Source: CAD feature listing. Evaluate the final solid. Frame: model axes, mm. A direction names the side the tool comes from. Round coordinates to 2 decimals unless told otherwise and drop trailing zeros. Write each loop counter-clockwise with the first axis right and the second up, starting at its lowest first coordinate (ties: lowest second). Pieces come first, ordered by that corner, then holes. Notation, with made-up numbers: M -22,-28.5 L -6,-28.5 A15 cw -6,-16.5 Z; hole C 88,49 d2. An arc over 180 degrees is marked long. Put each result on its own line as item: value. Start each with the question number.
```python
from build123d import *

# Parameters (mm, degrees)
SKETCH_1_R      = 1.7
EXTRUDE_1_DEPTH = 10
EXTRUDE_2_DEPTH = 1.3
FILLET_1_R      = 0.3
FILLET_2_R      = 0.3
SKETCH_3_R      = 1
EXTRUDE_3_DEPTH = 5
FILLET_3_R      = 2
SKETCH_4_W      = 3.4
SKETCH_4_H      = 10
EXTRUDE_4_DEPTH = 0.6


with BuildPart() as part:
    # 草圖1 → 填料-伸長1 (new body)
    with BuildSketch(Plane(origin=(0, 0, 0), x_dir=(1, 0, 0), z_dir=(0, 1, 0))):
        Polygon((13.5, -0.8), (11.5, -0.8), (11.5, -4.2), (13.5, -4.2), (13.5, -5), (0, -5), (-2.5, -5), (-2.5, 0), (0, 0), (13.5, 0), align=None)
        with Locations(Location((0, -2.5, 0), (0, 0, 270))):
            Circle(SKETCH_1_R, mode=Mode.SUBTRACT)
    extrude(amount=EXTRUDE_1_DEPTH)

    # 草圖2 → 填料-伸長2 (add)
    with BuildSketch(Plane(origin=(11.5, 0, 0), x_dir=(0, 0, -1), z_dir=(1, 0, 0))):
        Polygon((-4.2, 7.155796618), (-0.8, 5.655796618), (-0.8, 5), (-4.2, 6.5), align=None)
        Polygon((-4.2, 4.155796618), (-0.8, 2.655796618), (-0.8, 2), (-4.2, 3.5), align=None)
    extrude(amount=EXTRUDE_2_DEPTH)

    # 圓角1
    fillet_1_edges = [part.edges().sort_by_distance(p)[0] for p in [
        (12.8, 6.405796618, 2.5),
        (12.8, 5.75, 2.5),
        (12.8, 3.405796618, 2.5),
        (12.8, 2.75, 2.5),
    ]]
    fillet(fillet_1_edges, radius=FILLET_1_R - 0.0001)  # a hair under: the kernel refuses the full size

    # 圓角2
    fillet_2_edges = [part.edges().sort_by_distance(p)[0] for p in [
        (13.5, 5, 0),
        (13.5, 5, 0.8),
        (13.5, 5, 4.2),
        (13.5, 5, 5),
    ]]
    fillet(fillet_2_edges, radius=FILLET_2_R)

    # 草圖3 → 填料-伸長3 (add)
    with BuildSketch(Plane.XY):
        with BuildLine():
            Line((4.5, 10), (4.5, 15))
            ThreePointArc((4.5, 15), (7, 17.5), (9.5, 15))
            Line((9.5, 15), (9.5, 10))
            Line((9.5, 10), (4.5, 10))
        make_face()
        with Locations(Location((7, 15, 0), (0, 0, 180))):
            Circle(SKETCH_3_R, mode=Mode.SUBTRACT)
    extrude(amount=EXTRUDE_3_DEPTH)

    # 圓角3
    fillet_3_edges = [part.edges().sort_by_distance(p)[0] for p in [
        (-2.5, 5, 5),
        (-2.5, 5, 0),
    ]]
    fillet(fillet_3_edges, radius=FILLET_3_R)

    # 草圖4 → 填料-伸長4 (add)
    with BuildSketch(Plane(origin=(11.5, 0, 0), x_dir=(0, 0, -1), z_dir=(1, 0, 0))):
        with Locations((-2.5, 5)):
            Rectangle(SKETCH_4_W, SKETCH_4_H)
    extrude(amount=EXTRUDE_4_DEPTH)


solid = part.part
```
(1) Section query D-D (z = 3.55). Count the separate pieces of the cut face and the enclosed holes in it, and give its area (3 significant figures).
(2) Pull-direction query (Z, two-part tool) for faces 4 (the flat face through (12.3, 2.74, 2.48)), 5 (the flat face through (11, 10, 2)), 6 (the cylindrical face through (-1.9, 5.07, 0.57)); classes: +Z half, -Z half, draft (parallel to the pull), parting line (faces both ways), or undercut.
(3) Ray query, line 1 along X through (y, z) = (4.5, 2.5); line 2 along Y through (x, z) = (7, 2.8); line 3 along X through (y, z) = (15, 2.15). Return the intervals inside material, ascending.
(4) Section query C-C (y = 14.75). Return loops of the section in (x, z).
(5) Section query A-A (y = 8). Return loops of the section in (x, z), and give its area (3 significant figures).
(6) Section query B-B (x = 7). Return loops of the section in (y, z).
(7) Contact query for flat-ended pins moving along their axis: P1, Ø1.5, axis at y = 14.5, z = 1.5, coming from the +X side; P2, Ø1.5, axis at y = 12.5, z = 3.5, coming from the -X side; P3, Ø2.5, axis at x = 0, z = 2.5, coming from the -Y side; P4, Ø1, axis at y = 8.5, z = 2, coming from the +X side. Output: stop coordinate, or through.
(8) Access query for faces 1 (the flat face through (12.297, 6.416, 2.524)), 2 (the flat face through (12.1, 1, 3)), 3 (the flat face through (12.3, 5.74, 2.48)). Directions: +Z, -Z, +X, -X, +Y, -Y. A direction counts if a zero-diameter tool reaches every point of the face in a straight line with its end or side. Return the directions, or none.
Entries:
1. separate pieces: 2
1. enclosed holes: 1
1. area: 151 mm2
2. face 4: undercut
2. face 5: draft
2. face 6: -Z half
3. line 1: -2.5 to -1.7, 1.7 to 12.1
3. line 2: 0 to 14, 16 to 17.5
3. line 3: 4.5 to 6, 8 to 9.5
4. outline: M 4.5,0 L 6.03,0 L 6.03,5 L 4.5,5 Z; M 7.97,0 L 9.5,0 L 9.5,5 L 7.97,5 Z
5. outline: M -2.5,2 A2 ccw -0.5,0 L 13.2,0 A0.3 ccw 13.5,0.3 L 13.5,0.5 A0.3 ccw 13.2,0.8 L 12.1,0.8 L 12.1,4.2 L 13.2,4.2 A0.3 ccw 13.5,4.5 L 13.5,4.7 A0.3 ccw 13.2,5 L -0.5,5 A2 ccw -2.5,3 Z; hole C 0,2.5 d3.4
5. area: 64.4 mm2
6. outline: M 0,0 L 14,0 L 14,5 L 0,5 Z; M 16,0 L 17.5,0 L 17.5,5 L 16,5 Z
7. P1: x = 9.5
7. P2: x = 4.5
7. P3: through
7. P4: x = 12.1
8. face 1: +X, +Y
8. face 2: +X, -Y
8. face 3: +X
